Autodesk Inventor part; units mm, degrees
ref_plane "YZ Plane" through (0, 0, 0) normal (1, 0, 0) x (0, 1, 0)
ref_plane "XZ Plane" through (0, 0, 0) normal (0, 1, 0) x (-1, 0, 0)
sketch "草图1" plane through (0, 0, 0) normal (0, 1, 0) x (-1, 0, 0)
  circle A0 centre (0, 0) radius 10.3
  circle A1 centre (0, 0) radius 13
  line L0 (2.55, 6.35) -> (-2.55, 6.35)
  line L1 (-2.55, 6.35) -> (-2.55, -6.35)
  line L2 (-2.55, -6.35) -> (2.55, -6.35)
  line L3 (2.55, -6.35) -> (2.55, 6.35)
  line L4 (2.55, 6.35) -> (-2.55, -6.35) construction
  line L5 (-2.55, 6.35) -> (2.55, -6.35) construction
  line L6 (13, 13) -> (-13, 13)
  line L7 (-13, 13) -> (-13, -13)
  line L8 (-13, -13) -> (13, -13)
  line L9 (13, -13) -> (13, 13)
  line L10 (13, 13) -> (-13, -13) construction
  line L11 (-13, 13) -> (13, -13) construction
  point P0 (13, 0)
  point P1 (0, 13)
  point P2 (-13, 0)
  dimension "d0" = 20.6
  dimension "d1" = 26
  dimension "d2" = 5.1
  dimension "d3" = 12.7
extrude "拉伸1" add sketch "草图1" along normal blind 6 contours A0
extrude "拉伸2" add sketch "草图1" along normal blind 30 contours A1
ref_plane "工作平面1" through (0, 0, 13) normal (0, 0, 1) x (1, 0, 0)
sketch "草图2" plane through (0, 0, 13) normal (0, 0, 1) x (1, 0, 0)
  line L0 (-10.3, 30) -> (10.3, 30)
  circle A0 centre (0, 30) radius 1.4
  line L1 (0, 30) -> (0, 46.3)
  line L2 (0, 30) -> (0, 13.7)
  circle A1 centre (0, 13.7) radius 0.6
  circle A2 centre (0, 46.3) radius 0.6
  line L3 (0, 30) -> (16.3, 30)
  line L4 (0, 30) -> (-16.3, 30)
  line L5 (13, 30) -> (-13, 30)
  circle A3 centre (16.3, 30) radius 0.6
  circle A4 centre (-16.3, 30) radius 0.6
  line L6 (19.799, 30) -> (0, 10.201)
  line L7 (0, 10.201) -> (-19.799, 30)
  line L8 (-19.799, 30) -> (0, 49.799)
  line L9 (0, 49.799) -> (19.799, 30)
  line L10 (-14, 44) -> (14, 16) construction
  line L11 (14, 44) -> (-14, 16) construction
  point P0 (0, 0)
  dimension "d9" = 2.8
  dimension "d10" = 16.3
  dimension "d11" = 16.3
  dimension "d12" = 1.2
  dimension "d13" = 1.2
  dimension "d14" = 16.3
  dimension "d15" = 16.3
  dimension "d16" = 1.2
  dimension "d17" = 1.2
  dimension "d20" = 28
  dimension "d21" = 28
extrude "拉伸3" add sketch "草图1" along normal blind 50 contours A1 | A1 L6 L9 | A1 L7 L6
extrude "拉伸4" add sketch "草图2" against normal blind 2.7
extrude "拉伸5" cut sketch "草图2" against normal blind 10 contours A2
extrude "拉伸6" cut sketch "草图2" against normal blind 10 contours A1
equation "\"折弯半径\" = 厚度"
equation "\"最小余量\" = 2 * 厚度"
equation "\"过渡半径\" = 折弯半径"
equation "\"间隙大小\" = 厚度"
equation "\"折弯释压宽度\" = 厚度"
equation "\"折弯释压深度\" = 0.5 * 厚度"
equation "\"拐角释压尺寸\" = 4 * 厚度"
equation "\"Jacobi半径尺寸\" = 折弯半径"
properties part number "固定件"
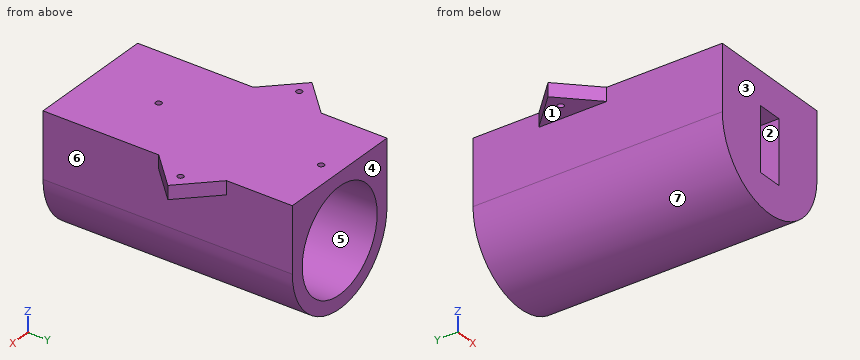
The listing builds one solid part. Answer for the finished solid, in the listing's coordinates (mm). Face numbers are marked on the shaded views. A direction names the side the tool comes from. Give positions to 0.01 mm unless a question says otherwise; leave off trailing zeros. Loops run counter-clockwise (first coordinate to the right, second up) from the corner with the lowest first, then second, coordinate; pieces in that order, holes last. Notation, with made-up numbers: M -31.75,-28.75 L 6.25,-28.75 A29 ccw 6.25,0.25 Z; hole C 31,-18.5 d7. An arc over 180 degrees is marked long. One line per item, written item: value.
Q1. A cutting plane is placed at B-B on y = 37.5. Determine the outline of the cut face in (x, z), then the cut area to 3 significant figures.
Working result:
outline: M -13,0 A13 ccw 13,0 L 13,13 L -13,13 Z; hole C 0,0 d20.6
area: 270 mm^2
Q2. For the marked faces 1, 2 and 3, determine the directions among +Z, -Z, +X, -X, +Y, -Y from which every point of the face is accessible in a straight line to the end or side of a thin tool.
Working result:
face 1: -Z, -X, +Y, -Y
face 2: +Y, -Y
face 3: +Z, -Z, +X, -X, -Y
Q3. Find the intervals of material crossed by line 1 (Y direction, x = 0, z = 11.85); line 2 (X direction, y = 25.5, z = -0.5); line 3 (Z direction, x = 0.5, y = 27.5), in increasing order. Write a range as from..to.
Working result:
line 1: y = 0..13.1, 14.3..45.7, 46.9..50
line 2: x = -12.99..-10.29, 10.29..12.99
line 3: z = -12.99..-10.29, 10.29..13
Q4. A cutting plane is placed at D-D on y = 13.7. Determine the outline of the cut face in (x, z), then the cut area to 3 significant figures.
Working result:
outline: M -13,0 A13 ccw 13,0 L 13,13 L 0.6,13 L 0.6,10.28 A10.3 cw long -0.6,10.28 L -0.6,13 L -13,13 Z
area: 267 mm^2
Q5. A cutting plane is placed at A-A on x = 0. Determine the outline of the cut face in (y, z), then the cut area to 3 significant figures.
Working result:
outline: M 0,-13 L 50,-13 L 50,-10.3 L 6,-10.3 L 6,-6.35 L 0,-6.35 Z; M 0,6.35 L 6,6.35 L 6,10.3 L 13.1,10.3 L 13.1,13 L 0,13 Z; M 14.3,10.3 L 45.7,10.3 L 45.7,13 L 14.3,13 Z; M 46.9,10.3 L 50,10.3 L 50,13 L 46.9,13 Z
area: 311 mm^2
Q6. A cutting plane is placed at C-C on z = -5.75. Determine the outline of the cut face in (x, y), then the cut area to 3 significant figures.
Working result:
outline: M -11.66,0 L -2.55,0 L -2.55,6 L -8.55,6 L -8.55,50 L -11.66,50 Z; M 2.55,0 L 11.66,0 L 11.66,50 L 8.55,50 L 8.55,6 L 2.55,6 Z
area: 383 mm^2
Q7. Flat-ended cylindrical pins translate along their axes: P1, Ø1.8, axis at y = 4.5, z = -3, coming from the -X side; P2, Ø4, axis at x = 15, z = -5.5, coming from the -Y side; P3, Ø1.5, axis at x = 1, y = 3.5, coming from the -Z side; P4, Ø5.5, axis at x = -18, y = 31, coming from the -Z side. Find the tip coordinate at first contact, or state that the pin passes through.
Working result:
P1: stops at x = -12.83
P2: passes through
P3: stops at z = -13
P4: stops at z = 10.3
Q8. Determine the mould class of the marked faces 4, 5, 6 and 7 for opening direction X: +X half, -X half, draft (parallel to the pull), parting line (faces both ways), or undercut.
Working result:
face 4: draft
face 5: undercut
face 6: +X half
face 7: parting line
